Geometry check sheet. Reference: the model listing, model coordinates, mm. Face numbers are marked on the shaded views. A direction names the side the tool comes from. Give positions to 0.01 mm unless a question says otherwise; leave off trailing zeros. Loops run counter-clockwise (first coordinate to the right, second up) from the corner with the lowest first, then second, coordinate; pieces in that order, holes last. Notation, with made-up numbers: (73, 32) -> (113, 32) arc R20 cw to (113, 42) -> close; hole circle Ø11 at (-19.5, 10). An arc over 180 degrees is marked (long way). One line per item, written item: value. Start each with the question number.
(1) Scan lines: line 1 along X through (y, z) = (-9, -3.5); line 2 along X through (y, z) = (-24, -4.25); line 3 along Z through (x, y) = (-0.5, -16). Record each from-to range of solid material in increasing order. Write a range as from..to.
(2) Sectioned sample at C-C, the plane y = -7. Record the cut outline in (x, z).
(3) Sectioned sample at D-D, the plane y = -11. Record the cut outline in (x, z).
(4) Tool access check on the marked faces 1, 2 and 3. Record the directions out of +Z, -Z, +X, -X, +Y, -Y that give a thin tool (end or side, any length) a straight path to the whole face; none if there is none.
(5) Draft check along Z on the marked faces 4, 5, 6 and 7. Enter one of: pulls with the +Z half, pulls with the -Z half, needs draft (parallel to the pull), parting line crosses it, or undercut.
(6) Sectioned sample at A-A, the plane z = -0.5. Record the cut outline in (x, y), then the cut area to 3 significant figures.
(7) Gauge pin test, flat ends, axial feed: pin 1 Ø5 at (y, z) = (-7, -2.5) entering from -X; pin 2 Ø3.5 at (y, z) = (-12.5, 1) entering from +X; pin 3 Ø1.2 at (x, y) = (0.5, -6.5) entering from +Z; pin 4 Ø1.5 at (x, z) = (-1.5, 1) entering from -Y. Record the tip position at first contact, or that the pin passes through.
(8) Sectioned sample at B-B, the plane x = 0. Record the cut outline in (y, z), then the cut area to 3 significant figures.
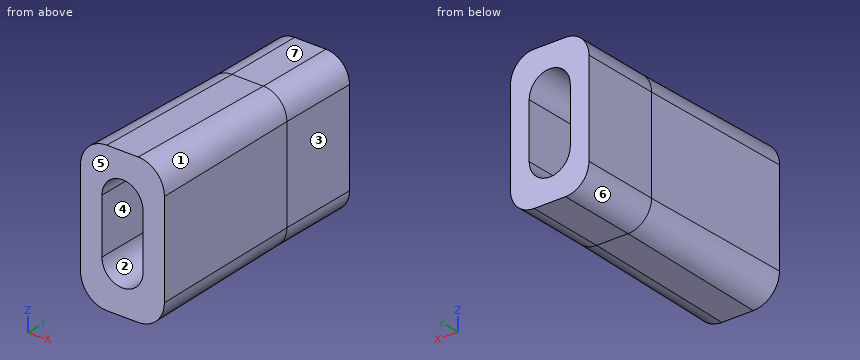
from build123d import *

# Parameters (mm, degrees)
BOSS_EXTRUDE1_DEPTH = 30
CUT_EXTRUDE2_REACH  = 33.718


with BuildPart() as part:
    # Sketch1 → Boss-Extrude1 (new body)
    with BuildSketch(Plane(origin=(0, 0, 0), x_dir=(1, 0, 0), z_dir=(0, 1, 0))):
        with BuildLine():
            Line((-2, -9), (2, -9))
            ThreePointArc((2, -9), (4.121320344, -8.121320344), (5, -6))
            Line((5, -6), (5, 6))
            ThreePointArc((5, 6), (4.121320344, 8.121320344), (2, 9))
            Line((2, 9), (-2, 9))
            ThreePointArc((-2, 9), (-4.121320344, 8.121320344), (-5, 6))
            Line((-5, 6), (-5, -6))
            ThreePointArc((-5, -6), (-4.121320344, -8.121320344), (-2, -9))
        make_face()
    extrude(amount=-BOSS_EXTRUDE1_DEPTH)

    # Sketch5 → Cut-Extrude2 (cut, up to next)
    with BuildSketch(Plane(origin=(0, 0, 0), x_dir=(1, 0, 0), z_dir=(0, 1, 0)), mode=Mode.PRIVATE) as cut_extrude2_sk1:
        with BuildLine():
            Line((-2.62, -3.5), (-2.62, 3.5))
            ThreePointArc((-2.62, 3.5), (0, 6.12), (2.62, 3.5))
            Line((2.62, 3.5), (2.62, -3.5))
            ThreePointArc((2.62, -3.5), (0, -6.12), (-2.62, -3.5))
        make_face()
    cut_extrude2_tool1 = extrude(cut_extrude2_sk1.sketch, amount=-CUT_EXTRUDE2_REACH, mode=Mode.PRIVATE) & part.part
    add(cut_extrude2_tool1.solids().sort_by_distance((0, 0, 0))[0], mode=Mode.SUBTRACT)

    # Sweep1: sweep along a path in Sketch1<3>
    with BuildLine(Plane(origin=(0, 0, 0), x_dir=(1, 0, 0), z_dir=(0, 1, 0))) as sweep1_path:
        Line((-2, -9), (2, -9))
        ThreePointArc((2, -9), (4.121320344, -8.121320344), (5, -6))
        Line((5, -6), (5, 6))
        ThreePointArc((5, 6), (4.121320344, 8.121320344), (2, 9))
        Line((2, 9), (-2, 9))
        ThreePointArc((-2, 9), (-4.121320344, 8.121320344), (-5, 6))
        Line((-5, 6), (-5, -6))
        ThreePointArc((-5, -6), (-4.121320344, -8.121320344), (-2, -9))
    # Sketch6 → Sweep1 (sweep)
    with BuildSketch(Plane.XY):
        Polygon((5, -10), (5.349101299, -30), (5, -30), align=None)
    sweep(path=sweep1_path.line)


solid = part.part
Calculated:
1. line 1: x = -5..-2.62, 2.62..5
1. line 2: x = -5.24..-2.51, 2.51..5.24
1. line 3: z = -9.1..-6.07, 6.07..9.1
2. outline: (-5, -6) arc R3 ccw to (-2, -9) -> (2, -9) arc R3 ccw to (5, -6) -> (5, 6) arc R3 ccw to (2, 9) -> (-2, 9) arc R3 ccw to (-5, 6) -> close; hole (-2.62, -3.5) arc R2.62 ccw to (2.62, -3.5) -> (2.62, 3.5) arc R2.62 ccw to (-2.62, 3.5) -> close
3. outline: (-5.02, -6) arc R3.02 ccw to (-2, -9.02) -> (2, -9.02) arc R3.02 ccw to (5.02, -6) -> (5.02, 6) arc R3.02 ccw to (2, 9.02) -> (-2, 9.02) arc R3.02 ccw to (-5.02, 6) -> close; hole (-2.62, -3.5) arc R2.62 ccw to (2.62, -3.5) -> (2.62, 3.5) arc R2.62 ccw to (-2.62, 3.5) -> close
4. face 1: +Z, +X, +Y
4. face 2: +Y, -Y
4. face 3: +Z, -Z, +X, +Y
5. face 4: undercut
5. face 5: needs draft
5. face 6: pulls with the -Z half
5. face 7: pulls with the +Z half
6. outline: (-5.35, -30) -> (-2.62, -30) -> (-2.62, 0) -> (-5, 0) -> (-5, -10) -> close; (2.62, -30) -> (5.35, -30) -> (5, -10) -> (5, 0) -> (2.62, 0) -> close
6. area: 150 mm2
7. pin 1: stops at x = -5
7. pin 2: stops at x = 5.07
7. pin 3: stops at z = 9
7. pin 4: passes through
8. outline: (-30, -9.35) -> (-10, -9) -> (0, -9) -> (0, -6.12) -> (-30, -6.12) -> close; (-30, 6.12) -> (0, 6.12) -> (0, 9) -> (-10, 9) -> (-30, 9.35) -> close
8. area: 180 mm2
